from build123d import *

# Parameters (mm, degrees)
BOSS_EXTRUDE1_DEPTH = 33
SKETCH2_R           = 2.2
CUT_EXTRUDE1_DEPTH  = 46.664537663
SKETCH3_R           = 2.5
BOSS_EXTRUDE2_DEPTH = 14


with BuildPart() as part:
    # Sketch1 → Boss-Extrude1 (new, symmetric)
    with BuildSketch(Plane.XY):
        with BuildLine():
            Line((12.5, -8), (24, -8))
            Line((24, -8), (24, -11.5))
            Line((24, -11.5), (-24, -11.5))
            Line((-24, -11.5), (-24, -8))
            Line((-24, -8), (-12.5, -8))
            Line((-12.5, -8), (-12.5, 0))
            ThreePointArc((-12.5, 0), (0, 12.5), (12.5, 0))
            Line((12.5, 0), (12.5, -8))
        make_face()
    extrude(amount=BOSS_EXTRUDE1_DEPTH, both=True)

    # Sketch2 → Cut-Extrude1 (cut, through all)
    with BuildSketch(Plane(origin=(0, -8, 0), x_dir=(1, 0, 0), z_dir=(0, 1, 0))):
        with Locations(Location((-18.5, 17.5, 0), (0, 0, 270))):
            Circle(SKETCH2_R)
        with Locations(Location((-18.5, -17.5, 0), (0, 0, 270))):
            Circle(SKETCH2_R)
        with Locations(Location((18.5, -17.5, 0), (0, 0, 270))):
            Circle(SKETCH2_R)
        with Locations(Location((18.5, 17.5, 0), (0, 0, 270))):
            Circle(SKETCH2_R)
    extrude(amount=-CUT_EXTRUDE1_DEPTH, mode=Mode.SUBTRACT)

    # Sketch3 → Boss-Extrude2 (add)
    with BuildSketch(Plane.XY.offset(33)):
        Circle(SKETCH3_R)
    boss_extrude2 = extrude(amount=BOSS_EXTRUDE2_DEPTH)

    # Mirror5: Boss-Extrude2 across plane
    add(boss_extrude2.mirror(Plane.XY))


solid = part.part
Model file for the job. Use its own axes, mm. A direction names the side the tool comes from. Coordinates: 2 decimals unless noted, no trailing zeros. Write each loop counter-clockwise with the first axis right and the second up, starting at its lowest first coordinate (ties: lowest second). Pieces come first, ordered by that corner, then holes. Notation, with made-up numbers: (-12.5, 20) -> (-7.5, 20) arc R35 cw to (-7.5, 52) -> close; hole circle Ø2 at (61, 26.25). An arc over 180 degrees is marked (long way). One line per item, written item: value. Start each with the question number.
1) Flat gauge pins, fed straight in: pin 1 Ø5 at (x, z) = (-8.5, 27) entering from +Y; pin 2 Ø9 at (y, z) = (-2.5, 6.5) entering from -X; pin 3 Ø3.5 at (x, z) = (16, -8.5) entering from +Y; pin 4 Ø3.5 at (x, z) = (18.5, 17.5) entering from +Y (3 decimals). Where does each tip first touch, or does it go through?
2) Probe probe 1 along X at (y, z) = (-9.7, 17.5); probe 2 along Y at (x, z) = (-16, 24); probe 3 along X at (y, z) = (-2.5, 13). List the from-to ranges inside material, lowest first.
3) Slice it at B-B on x = -18.5. Write the cut outline in (y, z), then the cut area to 3 significant figures.
4) Slice it at C-C on x = 0. Write the cut outline in (y, z).
5) Slice it at D-D on z = -29. Write the cut outline in (x, y).
6) Which spindle directions (+Z, -Z, +X, -X, +Y, -Y) get a long thin tool onto all of the face, cutting with end or side? Do faces 1 (the face through (-0.54, -2.44, -39.9)), 2 (the face through (-0.54, -2.44, 39.9)), 3 (the face through (12.5, -4, 0)). Say none if no direction does.
7) Pull direction X, two halves, no side cores. Call faces 4 (the face through (-24, -10, 0)), 5 (the face through (-19.343, -9.726, 19.532)), 6 (the face through (24, -10, 0)): +X half, -X half, draft (parallel to the pull), parting line (faces both ways), or undercut.
8) Slice it at A-A on z = -17.5. Write the cut outline in (x, y), then the cut area to 3 significant figures.
Answers follow:
1. pin 1: y = 10.97
1. pin 2: x = -12.5
1. pin 3: y = -8
1. pin 4: through
2. probe 1: -24 to -20.7, -16.3 to 16.3, 20.7 to 24
2. probe 2: -11.5 to -8
2. probe 3: -12.5 to 12.5
3. outline: (-11.5, -33) -> (-8, -33) -> (-8, -19.7) -> (-11.5, -19.7) -> close; (-11.5, -15.3) -> (-8, -15.3) -> (-8, 15.3) -> (-11.5, 15.3) -> close; (-11.5, 19.7) -> (-8, 19.7) -> (-8, 33) -> (-11.5, 33) -> close
3. area: 200 mm2
4. outline: (-11.5, -33) -> (-2.5, -33) -> (-2.5, -47) -> (2.5, -47) -> (2.5, -33) -> (12.5, -33) -> (12.5, 33) -> (2.5, 33) -> (2.5, 47) -> (-2.5, 47) -> (-2.5, 33) -> (-11.5, 33) -> close
5. outline: (-24, -11.5) -> (24, -11.5) -> (24, -8) -> (12.5, -8) -> (12.5, 0) arc R12.5 ccw to (-12.5, 0) -> (-12.5, -8) -> (-24, -8) -> close
6. face 1: -Z
6. face 2: +Z
6. face 3: +Z, -Z, +X, +Y
7. face 4: -X half
7. face 5: undercut
7. face 6: +X half
8. outline: (-24, -11.5) -> (-20.7, -11.5) -> (-20.7, -8) -> (-24, -8) -> close; (-16.3, -11.5) -> (16.3, -11.5) -> (16.3, -8) -> (12.5, -8) -> (12.5, 0) arc R12.5 ccw to (-12.5, 0) -> (-12.5, -8) -> (-16.3, -8) -> close; (20.7, -11.5) -> (24, -11.5) -> (24, -8) -> (20.7, -8) -> close
8. area: 583 mm2
